Read the model definition and answer for the solid it produces. Units are mm, in the model's axes. A direction names the side the tool comes from. Coordinates: 2 decimals unless noted, no trailing zeros. Loops run counter-clockwise (first coordinate to the right, second up) from the corner with the lowest first, then second, coordinate; pieces in that order, holes last. Notation, with made-up numbers: M 45,-6.75 L 86,-6.75 A21 cw 86,23.25 Z; hole C -36.5,-31.75 d10. An arc over 180 degrees is marked long. Put each result on its own line as item: value.
from build123d import *

# Parameters (mm, degrees)
SALIENTE_EXTRUIR1_DEPTH = 103
CROQUIS2_W              = 10
CROQUIS2_H              = 6
SALIENTE_EXTRUIR2_DEPTH = 10
CROQUIS8_R              = 1.5
CORTAR_EXTRUIR3_DEPTH   = 214.213522317


with BuildPart() as part:
    # Croquis1 → Saliente-Extruir1 (new, symmetric)
    with BuildSketch(Plane(origin=(0, 0, 0), x_dir=(1, 0, 0), z_dir=(0, 1, 0))):
        Polygon((-40, 0), (40, 0), (63.334523779, 23.334523779), (68.991378029, 17.67766953), (43.313708499, -8), (-44.015502165, -8), (-66.132956944, 21.681064581), (-59.718117141, 26.46121419), align=None)
    extrude(amount=SALIENTE_EXTRUIR1_DEPTH, both=True)

    # Croquis2 → Saliente-Extruir2 (add)
    with BuildSketch(Plane(origin=(0, 0, 0), x_dir=(-1, 0, 0), z_dir=(0, 0, -1))):
        with Locations((29, -94)):
            Rectangle(CROQUIS2_W, CROQUIS2_H)
        with Locations((-29, -94)):
            Rectangle(CROQUIS2_W, CROQUIS2_H)
    extrude(amount=SALIENTE_EXTRUIR2_DEPTH)

    # Croquis8 → Cortar-Extruir3 (cut, through all)
    with BuildSketch(Plane.XZ.offset(97)):
        with Locations(Location((29, -5, 0), (0, 0, 270))):
            Circle(CROQUIS8_R)
        with Locations(Location((-29, -5, 0), (0, 0, 270))):
            Circle(CROQUIS8_R)
    extrude(amount=-CORTAR_EXTRUIR3_DEPTH, mode=Mode.SUBTRACT)


solid = part.part
1) Find section C-C, the plane z = 3. Write down the section's boundary in (x, y), plus the area to 3 significant figures.
Answer list:
outline: M -47.74,-103 L 48.31,-103 L 48.31,103 L -47.74,103 Z
area: 19,800 mm^2
2) Find section B-B, the plane x = -5. Write down the section's boundary in (y, z), plus the area to 3 significant figures.
Answer list:
outline: M -103,0 L 103,0 L 103,8 L -103,8 Z
area: 1,650 mm^2
3) Find section A-A, the plane y = 55. Write down the section's boundary in (x, z).
Answer list:
outline: M -66.13,-21.68 L -59.72,-26.46 L -40,0 L 40,0 L 63.33,-23.33 L 68.99,-17.68 L 43.31,8 L -44.02,8 Z
4) Which of the six approach directions +Z, -Z, +X, -X, +Y, -Y give full straight-line access (tool end or side, diameter ignored) to faces 1 (the flat face through (30.2, -97, -3.8)), 2 (the flat face through (0, 1, 8)), 3 (the flat face through (30.2, -91, -3.8)), 4 (the flat face through (66.12, 1.44, -20.55)), 5 (the flat face through (-50, 1.44, -13.42))?
Answer list:
face 1: -Z, -Y
face 2: +Z, +X, -X, +Y, -Y
face 3: -Z, +Y
face 4: -Z, +X, +Y, -Y
face 5: -Z, +Y, -Y
5) Given pin 1 Ø3.5 at (x, z) = (29, -5) entering from +Y; pin 2 Ø3.5 at (x, z) = (-29, -5) entering from -Y; pin 3 Ø3 at (x, y) = (-30, -95.5) entering from -Z, each flat-ended and moving along its own axis, determine where each tip first touches the part or whether it passes through.
Answer list:
pin 1: stops at y = -91
pin 2: stops at y = -97
pin 3: stops at z = -10
6) Straight lines are drawn through the part: line 1 (X direction, y = -95, z = -5); line 2 (Z direction, x = -7, y = 23); line 3 (X direction, y = 47, z = -14.5). For each, find the intervals that lie inside material, in ascending order. Write a range as [from, to].
Answer list:
line 1: x = [-53.7, -43.73], [-34, -30.5], [-27.5, -24], [24, 27.5], [30.5, 34], [45, 56.31]
line 2: z = [0, 8]
line 3: x = [-60.78, -50.8], [54.5, 65.81]
7) Determine the mould class of faces 6 (the flat face through (-54.919, 1.442, -6.633)), 7 (the flat face through (56.332, 1.442, -5.019)), 8 (the flat face through (24, -94, -5)) for opening direction X: released by +X, released by -X, zero draft, split by the parting line, or undercut.
Answer list:
face 6: released by -X
face 7: released by +X
face 8: undercut
